Autodesk Inventor part; units mm, degrees
ref_plane "Work Plane3" through (-49.05, -33.575, -1214.2) normal (0, -1, 0) x (1, 0, 0)
ref_plane "YZ Plane" through (0, 0, 0) normal (1, 0, 0) x (0, 1, 0)
ref_plane "XZ Plane" through (0, 0, 0) normal (0, 1, 0) x (-1, 0, 0)
sketch "Sketch1" plane through (0, 0, 0) normal (0, 1, 0) x (-1, 0, 0)
  line L0 (0, 0) -> (60, 0) construction
  line L1 (60, 0) -> (60, -20) construction
  line L2 (60, -20) -> (0, -20) construction
  line L3 (0, -20) -> (0, 0) construction
  line L4 (60.5, 0.5) -> (-0.5, 0.5)
  line L5 (-0.5, 0.5) -> (-0.5, -20.5)
  line L6 (-0.5, -20.5) -> (60.5, -20.5)
  line L7 (60.5, -20.5) -> (60.5, 0.5)
  circle A0 centre (53, -10) radius 2.5
  circle A1 centre (7, -10) radius 2.5
  line L8 (53, -10) -> (7, -10) construction
  point P0 (30, -10)
  point P1 (30, -20)
  point P2 (0, -10)
  dimension "d0" = 20
  dimension "d1" = 60
  dimension "d2" = 0.5
  dimension "d3" = 0.5
  dimension "d4" = 0.5
  dimension "d5" = 0.5
  dimension "d6" = 5
  dimension "d7" = 46
sketch "Sketch2" plane through (0, 0, 0) normal (0, 1, 0) x (-1, 0, 0)
  line L0 (-5.4, 5) -> (65.4, 5)
  line L1 (65.4, 5) -> (65.4, -25)
  line L2 (65.4, -25) -> (-5.4, -25)
  line L3 (-5.4, -25) -> (-5.4, 5)
  line L4 (60.5, -20.5) -> (60.5, 0.5) construction
  line L5 (-0.5, 0.5) -> (-0.5, -20.5) construction
  line L6 (-0.5, -20.5) -> (60.5, -20.5) construction
  point P0 (0, 0)
  point P1 (60.5, -10)
  point P2 (65.4, -10)
  point P3 (30, -20.5)
  point P4 (30, -25)
  dimension "d9" = 70.8
  dimension "d10" = 30
  dimension "d44" = 35.4
extrude "Extrusion1" add sketch "Sketch2" against normal blind 30.4
extrude "Extrusion3" cut sketch "Sketch1" against normal blind 43.3375 and the other way blind 30.4 contours A0 | A1
sketch "Sketch3" plane through (5.4, -30.4, -25) normal (0, 0, -1) x (1, 0, 0)
  line L0 (-70.8, 0) -> (0, 0)
  line L1 (0, 0) -> (0, 17.5)
  line L2 (0, 17.5) -> (-9.5, 17.5)
  line L3 (-9.5, 17.5) -> (-9.5, 5.08)
  line L4 (-14.58, 0) -> (-56.22, 0)
  line L5 (-61.3, 5.08) -> (-61.3, 17.5)
  line L6 (-61.3, 17.5) -> (-70.8, 17.5)
  line L7 (-70.8, 17.5) -> (-70.8, 0)
  arc A0 (-14.58, 0) -> (-9.5, 5.08) centre (-14.58, 5.08) ccw
  arc A1 (-61.3, 5.08) -> (-56.22, 0) centre (-56.22, 5.08) ccw
  point P0 (-9.5, 0)
  point P1 (-61.3, 0)
  point P2 (-61.3, 11.29)
  point P3 (-9.5, 11.29)
  point P4 (-4.75, 17.5)
  dimension "d94" = 51.8
  dimension "d95" = 17.5
  dimension "d96" = 5.08
extrude "Extrusion4" add sketch "Sketch3" against normal up to surface (30 mm away)
ref_plane "Work Plane3" through (-49.05, -33.575, -1214.2) normal (0, -1, 0) x (1, 0, 0)
sketch "Sketch4" plane through (0, 0, 0) normal (0, 1, 0) x (1, 0, 0)
  line L0 (-60.5, 20.5) -> (0.5, 20.5) construction
  line L1 (-60.5, -0.5) -> (-60.5, 20.5) construction
  circle A0 centre (-40, 10) radius 3
  line L2 (5.4, 25) -> (-65.4, 25)
  line L3 (-65.4, 25) -> (-65.4, -5)
  circle A1 centre (-20, 10) radius 3
  line L4 (-40, 10) -> (-20, 10) construction
  point P0 (0, 0)
  point P1 (-30, 20.5)
  point P2 (-60.5, 10)
  point P3 (-65.4, 20.5)
  point P4 (5.4, 20.5)
  point P5 (-30, 20.5)
  point P6 (-60.5, 10)
  point P7 (-65.4, 10)
  point P8 (-30, 25)
  point P9 (-30, 10)
  dimension "d82" = 6
  dimension "d98" = 20
extrude "Extrusion5" cut sketch "Sketch4" against normal up to surface (33.575 mm away)
extrude "Extrusion2" cut sketch "Sketch1" against normal blind 43.3375 and the other way blind 5 contours A0 | A1
sketch "Sketch8" plane through (15.4, 40, -25) normal (0, 0, -1) x (1, 0, 0)
  line L0 (25.4, 30) -> (34.4, 30)
  line L1 (34.4, 30) -> (35.4, 31)
  line L2 (35.4, 31) -> (35.4, 34)
  line L3 (35.4, 34) -> (31.95, 37.45)
  line L4 (31.95, 37.45) -> (31.95, 39.8767)
  line L5 (31.95, 39.8767) -> (33.1672, 41.0939)
  arc A0 (34.8792, 42.8058) -> (33.1672, 41.0939) centre (35.1489, 40.8241) ccw
  line L6 (34.8792, 42.8058) -> (35.4, 43.3267)
  line L7 (35.4, 43.3267) -> (35.4, 44.66)
  line L8 (35.4, 44.66) -> (34.8792, 45.1808)
  arc A1 (33.1672, 46.8928) -> (34.8792, 45.1808) centre (35.1489, 47.1626) ccw
  line L9 (33.1672, 46.8928) -> (32.56, 47.5)
  line L10 (32.56, 47.5) -> (25.4, 47.5)
  line L11 (25.4, 47.5) -> (25.4, 30) construction
  line L12 (33.1672, 41.0939) -> (34.8792, 42.8058) construction
  line L13 (33.1672, 46.8928) -> (34.8792, 45.1808) construction
  line L14 (25.4, 30) -> (16.4, 30)
  line L15 (16.4, 30) -> (15.4, 31)
  line L16 (15.4, 31) -> (15.4, 34)
  line L17 (15.4, 34) -> (18.85, 37.45)
  line L18 (18.85, 37.45) -> (18.85, 39.8767)
  line L19 (18.85, 39.8767) -> (17.6328, 41.0939)
  arc A2 (17.6328, 41.0939) -> (15.9208, 42.8058) centre (15.6511, 40.8241) ccw
  line L20 (15.9208, 42.8058) -> (15.4, 43.3267)
  line L21 (15.4, 43.3267) -> (15.4, 44.66)
  line L22 (15.4, 44.66) -> (15.9208, 45.1808)
  arc A3 (15.9208, 45.1808) -> (17.6328, 46.8928) centre (15.6511, 47.1626) ccw
  line L23 (17.6328, 46.8928) -> (18.24, 47.5)
  line L24 (18.24, 47.5) -> (25.4, 47.5)
  line L25 (17.6328, 41.0939) -> (15.9208, 42.8058) construction
  line L26 (17.6328, 46.8928) -> (15.9208, 45.1808) construction
  arc A4 (50.8, 26.825) -> (47.625, 30) centre (47.625, 26.825) ccw construction
  line L27 (34.4, 30) -> (35.4, 30)
  line L28 (3.175, 30) -> (47.625, 30)
  line L29 (35.4, 31) -> (35.4, 30)
  line L30 (15.4, 31) -> (15.4, 30)
  line L31 (15.4, 30) -> (16.4, 30)
  point P0 (-15.4, 40)
  point P1 (35.4, 32.5)
  dimension "d64" = 1
  dimension "d65" = 3
  dimension "d66" = 135
  dimension "d67" = 2
  dimension "d69" = 3.45
  dimension "d71" = 17.5
  dimension "d72" = 7.16
  dimension "d73" = 2.375
  dimension "d74" = 1.3333
  dimension "d75" = 2.4211
  dimension "d76" = 15.4
  dimension "d77" = 10
extrude "Extrusion8" [suppressed]
thicken "Thicken1" [suppressed]
sketch "Sketch11" plane through (0, 0, 0) normal (0, 1, 0) x (1, 0, 0)
  circle A0 centre (-20, 10) radius 6
  circle A1 centre (-40, 10) radius 3
  circle A2 centre (-20, 10) radius 3
  circle A3 centre (-40, 10) radius 6
  point P0 (0, 0)
  dimension "d99" = 12
extrude "Extrusion11" cut sketch "Sketch11" against normal blind 10 contours A0 | A1 | A2 | A3
chamfer "Chamfer1" distance 2 angle 45 12 edges at (5.4, 0, -10) (-30, 0, -25) (5.4, -23.95, -25) (-65.4, -23.95, -25) (-55.9, -47.9, -10) (5.4, -47.9, -10) (-30, 0, 5) (-65.4, 0, -10) (-65.4, -23.95, 5) (-65.4, -47.9, -10) (-4.1, -47.9, -10) (5.4, -23.95, 5)
properties part number "BK12_Spacer"
For this review, take the finished solid that the model builds, in its own axes (mm). A direction names the side the tool comes from. Round coordinates to 2 decimals unless told otherwise and drop trailing zeros. Write each loop counter-clockwise with the first axis right and the second up, starting at its lowest first coordinate (ties: lowest second). Pieces come first, ordered by that corner, then holes. Notation, with made-up numbers: (-25.5, 16.5) - (-21.5, 16.5) arc R27 ccw to (-21.5, 41.5) - close; hole circle Ø3 at (50, -38). An arc over 180 degrees is marked (long way). Put each result on its own line as item: value.
Q1. Machinability: for faces 4 (the face through (4.4, -46.9, -9.8)), 5 (the face through (-19, -10, -13)), 6 (the face through (-55.74, -34.22, -10.21)), which of the approach directions +Z, -Z, +X, -X, +Y, -Y give a long, thin tool a straight path to every point of the face, cutting with its end or side? Answer none if there is none.
Solved:
face 4: +Z, -Z, +X, -Y
face 5: +Y
face 6: +Z, -Z, -Y
Q2. We need section A-A (x = -20). Give the boundary of the cut face in (y, z).
Solved:
outline: (-30.4, -25) - (-2, -25) - (0, -23) - (0, -16) - (-10, -16) - (-10, -13) - (-30.4, -13) - close; (-30.4, -7) - (-10, -7) - (-10, -4) - (0, -4) - (0, 3) - (-2, 5) - (-30.4, 5) - close
Q3. We need section C-C (y = -11). Give the boundary of the cut face in (x, z), and give its area (3 significant figures).
Solved:
outline: (-65.4, -23) - (-63.4, -25) - (3.4, -25) - (5.4, -23) - (5.4, 3) - (3.4, 5) - (-63.4, 5) - (-65.4, 3) - close; hole circle Ø5 at (-53, -10); hole circle Ø6 at (-40, -10); hole circle Ø6 at (-20, -10); hole circle Ø5 at (-7, -10)
area: 2,020 mm2
Q4. Wall thickness on probe 1 along X at (y, z) = (-3, -10); probe 2 along X at (y, z) = (-21, -10); probe 3 along X at (y, z) = (-3, -14): over which ranges is each line inside the solid? List them lowest first.
Solved:
probe 1: x = -65.4 to -55.5, -50.5 to -46, -34 to -26, -14 to -9.5, -4.5 to 5.4
probe 2: x = -65.4 to -55.5, -50.5 to -43, -37 to -23, -17 to -9.5, -4.5 to 5.4
probe 3: x = -65.4 to -44.47, -35.53 to -24.47, -15.53 to 5.4
Q5. Mouldability with a two-part tool opening along X and no side actions: class faces 1 (the face through (-44.76, -4.93, -6.35)), 2 (the face through (-64.4, -25.3, 4)), 3 (the face through (-30, -20, -25)) as released by +X, released by -X, zero draft, split by the parting line, or undercut.
Solved:
face 1: undercut
face 2: released by -X
face 3: zero draft
Q6. We need section D-D (x = -10.5). Give the boundary of the cut face in (y, z), and give its area (3 significant figures).
Solved:
outline: (-30.4, -25) - (-2, -25) - (0, -23) - (0, 3) - (-2, 5) - (-30.4, 5) - close
area: 908 mm2
Q7. Insertion check: pin 1 Ø9.5 at (x, z) = (-20, -10) entering from +Y; pin 2 Ø4 at (x, z) = (-53, -10) entering from +Y; pin 3 Ø6 at (x, z) = (-41.5, -1.5) entering from -Y. Each pin has a flat end and moves straight along its axis. Give the tip position at first contact, or say it passes through.
Solved:
pin 1: stops at y = -10
pin 2: passes through
pin 3: stops at y = -30.4
Q8. We need section B-B (z = -19). Give the boundary of the cut face in (x, y).
Solved:
outline: (-65.4, -45.9) - (-63.4, -47.9) - (-57.9, -47.9) - (-55.9, -45.9) - (-55.9, -35.48) arc R5.08 cw to (-50.82, -30.4) - (-9.18, -30.4) arc R5.08 cw to (-4.1, -35.48) - (-4.1, -45.9) - (-2.1, -47.9) - (3.4, -47.9) - (5.4, -45.9) - (5.4, -2) - (3.4, 0) - (-63.4, 0) - (-65.4, -2) - close
